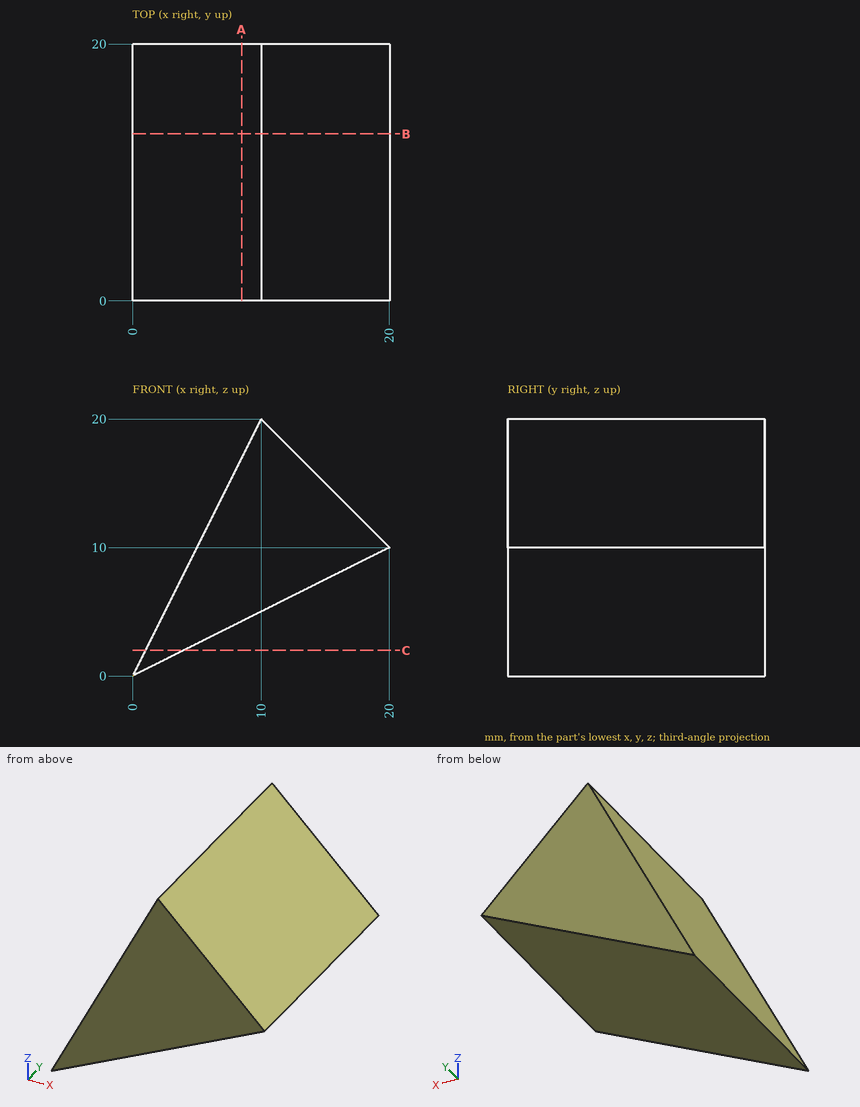
Print and shaded views of the part. All mm, measured from the part's lowest x, y and z. Give positions to 0.01 mm unless a question says otherwise; leave off trailing zeros. Loops run counter-clockwise (first coordinate to the right, second up) from the corner with the lowest first, then second, coordinate; pieces in that order, holes last. Notation, with made-up numbers: (29, 2) - (38, 2) arc R32 ccw to (38, 38) - close; hole circle Ø6 at (-6.75, 55.5). An arc over 180 degrees is marked (long way). Use a Markdown table: item, result.
(1) Wall check: line 1 along X through (y, z) = (7.75, 12.5); line 2 along X through (y, z) = (1.5, 14); line 3 along Z through (x, y) = (1, 9.75). Give the ranges that are in metal, low to high.
Taken from the geometry:
| item | result |
|---|---|
| line 1 | 6.25 to 17.5 |
| line 2 | 7 to 16 |
| line 3 | 0.5 to 2 |
(2) Band-saw the part on A-A (x = 8.5). Give the cut face in (y, z).
Taken from the geometry:
| item | result |
|---|---|
| outline | (0, 4.25) - (20, 4.25) - (20, 17) - (0, 17) - close |
(3) Drop flat-ended pins along their axis: pin 1 Ø2 at (y, z) = (17, 10.5) entering from -X; pin 2 Ø5 at (y, z) = (4, 15) entering from +X; pin 3 Ø4 at (x, y) = (9.5, 2.5) entering from +Z. Give the stop position or say it passes through.
Taken from the geometry:
| item | result |
|---|---|
| pin 1 | x = 4.75 |
| pin 2 | x = 17.5 |
| pin 3 | z = 20 |
(4) Band-saw the part on B-B (y = 13). Give the cut face in (x, z), and give its area (3 significant figures).
Taken from the geometry:
| item | result |
|---|---|
| outline | (0, 0) - (20, 10) - (10, 20) - close |
| area | 150 mm2 |
(5) Band-saw the part on C-C (z = 2). Give the cut face in (x, y), and give its area (3 significant figures).
Taken from the geometry:
| item | result |
|---|---|
| outline | (1, 0) - (4, 0) - (4, 20) - (1, 20) - close |
| area | 60.0 mm2 |
